The drawing under review shows one solid part. Ordinate dimensions are in mm from its lowest x, y, z. A direction names the side the tool comes from. Coordinates: 2 decimals unless noted, no trailing zeros. Loops run counter-clockwise (first coordinate to the right, second up) from the corner with the lowest first, then second, coordinate; pieces in that order, holes last. Notation, with made-up numbers: M 66,64.5 L 82,64.5 A10 ccw 82,71.5 Z; hole C -31.75,-33.75 d3. An arc over 180 degrees is marked long. Answer as a JSON object with one key per item and string values. Group by question number.
1. Consider section C-C (z = 2.15). State the section outline as (x, y) points (1 decimal), then the cut area to 3 significant figures.
2. To check wall thickness, follow probe 1 along Z at (x, y) = (8, 4.25); probe 2 along Y at (x, z) = (3, 1.1) (1 decimal); probe 3 along X at (y, z) = (6.75, 4.35) (1 decimal). State the ranges of each line that lie inside material, in increasing order.
3. Consider section D-D (y = 1.5). State the section outline as (x, z) points.
4. Consider section B-B (x = 5.75). State the section outline as (y, z) points (1 decimal).
5. Insertion check: pin 1 (5 mm diameter, centred on x = 10.68, y = 7, fed in from +Z); pin 2 (2 mm diameter, centred on x = 1.5, z = 3, fed in from -Y); pin 3 (5 mm diameter, centred on x = 11.5, y = 8, fed in from +Z); pin 4 (3 mm diameter, centred on x = 9.5, y = 4, fed in from -Z). Each pin has a flat end and moves straight along its axis. Give the tip position at first contact, or say it passes through.
6. Consider section A-A (z = 4.3). State the section outline as (x, y) points (1 decimal).
7. Draft analysis for pull direction Y (two halves, no side actions). For the marked faces 4, 5 and 6, state which applies: +Y half, -Y half, draft (parallel to the pull), parting line (faces both ways), or undercut.
8. Machinability: for the marked faces 1, 2 and 3, which of the approach directions +Z, -Z, +X, -X, +Y, -Y give a long, thin tool a straight path to every point of the face, cutting with its end or side? Answer none if there is none.
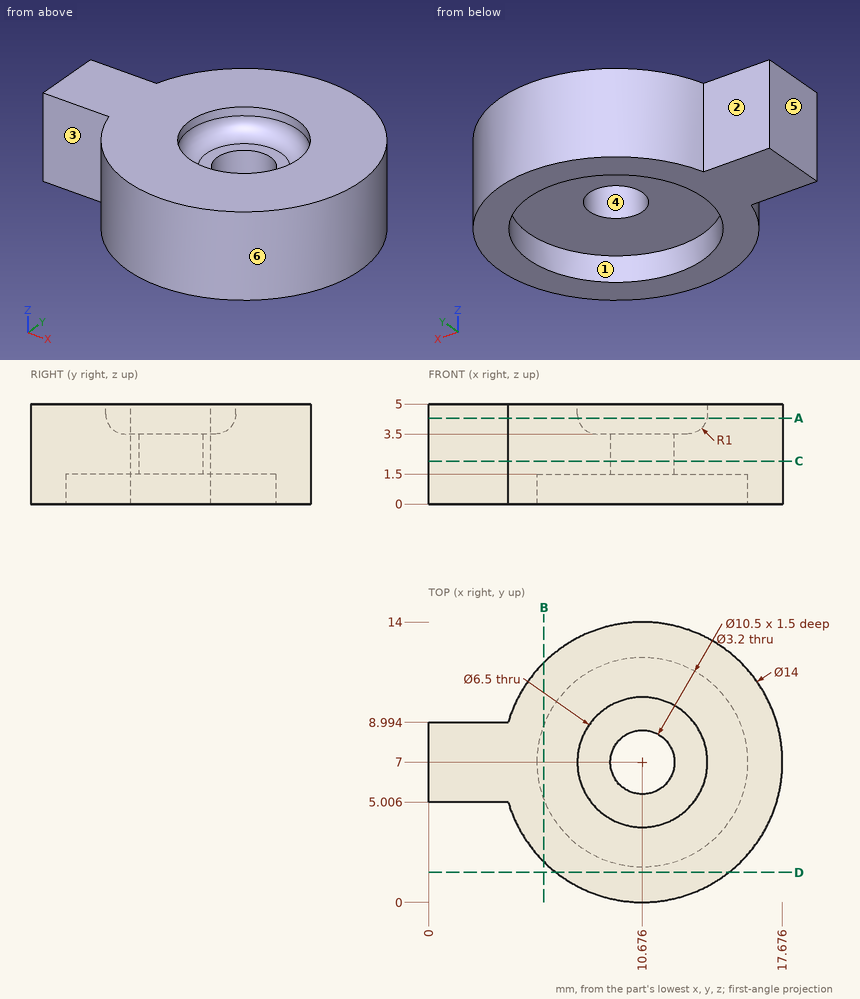
Findings below:
{
 "1": {"outline": "M 0,5 L 4,5 A7 ccw long 4,9 L 0,9 Z; hole C 10.7,7 d3.2", "area": "161 mm^2"},
 "2": {"probe 1": "z = 1.5 to 5", "probe 2": "y = 5 to 9", "probe 3": "x = 0 to 7.4, 13.9 to 17.7"},
 "3": {"outline": "M 6.35,0 L 15.01,0 L 15.01,5 L 6.35,5 Z"},
 "4": {"outline": "M 2,0 L 5.2,0 L 5.2,1.5 L 8.8,1.5 L 8.8,0 L 12,0 L 12,5 L 2,5 Z"},
 "5": {"pin 1": "stops at z = 3.53", "pin 2": "stops at y = 5.01", "pin 3": "stops at z = 5", "pin 4": "stops at z = 1.5"},
 "6": {"outline": "M 0,5 L 4,5 A7 ccw long 4,9 L 0,9 Z; hole C 10.7,7 d6.5"},
 "7": {"face 4": "undercut", "face 5": "draft", "face 6": "parting line"},
 "8": {"face 1": "-Z", "face 2": "+Z, -Z, -X, +Y", "face 3": "+Z, -Z, -X, -Y"}
}
